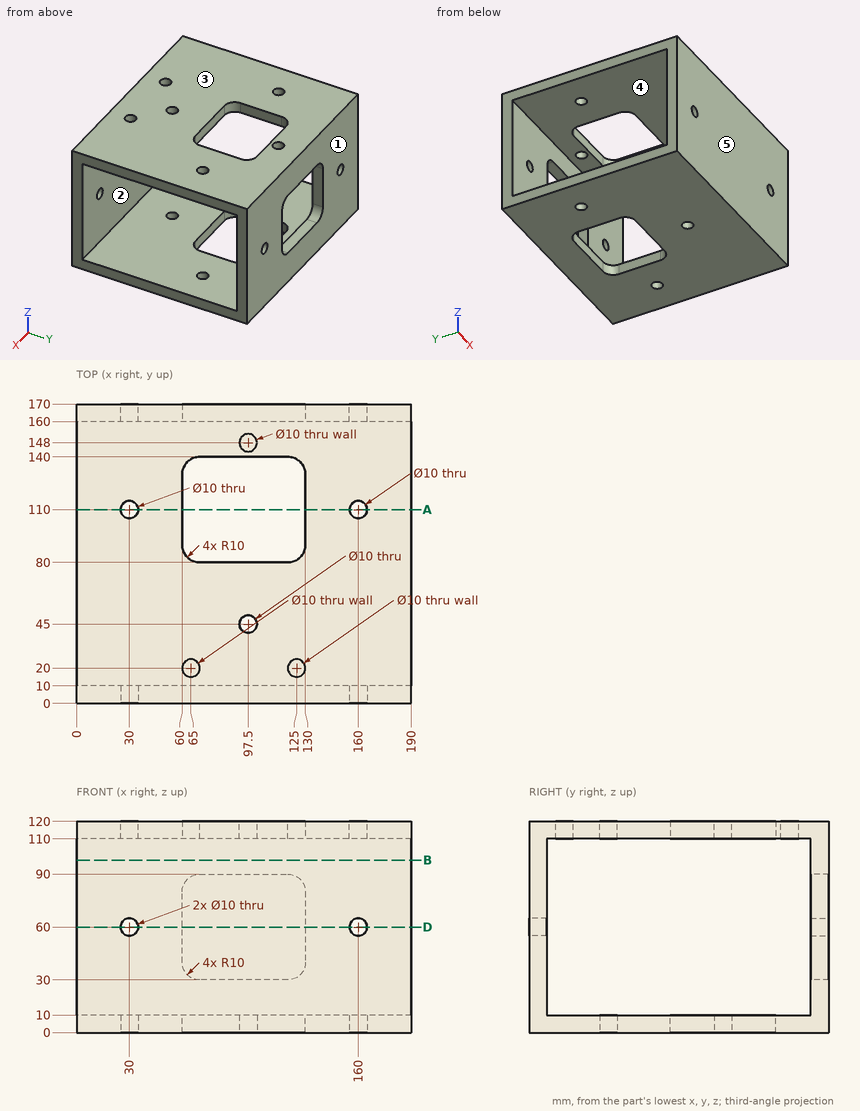
Print and shaded views of the part. All mm, measured from the part's lowest x, y and z. A direction names the side the tool comes from. Give positions to 0.01 mm unless a question says otherwise; leave off trailing zeros. Loops run counter-clockwise (first coordinate to the right, second up) from the corner with the lowest first, then second, coordinate; pieces in that order, holes last. Notation, with made-up numbers: (56.5, -40) - (80.5, -40) arc R30 cw to (80.5, -2) - close; hole circle Ø5 at (78.25, 77.5). An arc over 180 degrees is marked (long way). One line per item, written item: value. Start each with the question number.
1. Pin check, flat tip, straight feed: pin 1 (6 mm diameter, centred on x = 30, y = 110, fed in from -Z). Stop position of the tip, or through.
2. Slice it at A-A (y = 110). Give the number of separate pieces and of enclosed holes in the cut face, plus the area to 3 significant figures.
3. Slice it at D-D (z = 60). List the corners of the cut face in (x, y).
4. Slice it at B-B (z = 98). List the corners of the cut face in (x, y).
5. Which spindle directions (+Z, -Z, +X, -X, +Y, -Y) get a long thin tool onto all of the face, cutting with end or side? Do the marked faces 1 and 2. Say none if no direction does.
6. Pull direction Z, two halves, no side cores. Call the marked faces 3, 4 and 5: pulls with the +Z half, pulls with the -Z half, needs draft (parallel to the pull), parting line crosses it, or undercut.
7. Probe L1, parallel to Y at x = 97, z = 113; L2, parallel to X at y = 2, z = 60; L3, parallel to X at y = 167.75, z = 60. List the from-to ranges inside material, lowest first. Write a range as from..to.
Solution:
1. pin 1: passes through
2. separate pieces: 8
2. enclosed holes: 0
2. area: 2,000 mm^2
3. outline: (0, 0) - (25, 0) - (25, 10) - (0, 10) - close; (0, 160) - (25, 160) - (25, 170) - (0, 170) - close; (35, 0) - (155, 0) - (155, 10) - (35, 10) - close; (35, 160) - (60, 160) - (60, 170) - (35, 170) - close; (130, 160) - (155, 160) - (155, 170) - (130, 170) - close; (165, 0) - (190, 0) - (190, 10) - (165, 10) - close; (165, 160) - (190, 160) - (190, 170) - (165, 170) - close
4. outline: (0, 0) - (190, 0) - (190, 10) - (0, 10) - close; (0, 160) - (190, 160) - (190, 170) - (0, 170) - close
5. face 1: +Z, -Z, +X, -X, +Y
5. face 2: +X, -X
6. face 3: pulls with the +Z half
6. face 4: undercut
6. face 5: needs draft
7. L1: y = 0..40.03, 49.97..80, 140..143.03, 152.97..170
7. L2: x = 0..25, 35..155, 165..190
7. L3: x = 0..25, 35..60, 130..155, 165..190
